from build123d import *

# Parameters (mm, degrees)
SKETCH1_W               = 40
SKETCH1_H               = 20
BOSS_EXTRUDE1_DEPTH     = 4
SKETCH2_W               = 10
SKETCH2_H               = 20
BOSS_EXTRUDE2_DEPTH     = 10
SKETCH3_R               = 1.5
CUT_EXTRUDE1_DEPTH      = 20
SKETCH4_R               = 1.5
CUT_EXTRUDE2_DEPTH      = 20
CUT_EXTRUDE3_DEPTH      = 43.242250662
CUT_EXTRUDE3_DEPTH_BACK = 20
SKETCH6_W               = 40
SKETCH6_H               = 20
BOSS_EXTRUDE3_DEPTH     = 4.5
CUT_EXTRUDE5_DEPTH      = 4.5
CUT_EXTRUDE6_DEPTH      = 14.5
SKETCH9_W               = 40
SKETCH9_H               = 20
CUT_EXTRUDE7_DEPTH      = 1.5


with BuildPart() as part:
    # Sketch1 → Boss-Extrude1 (new body)
    with BuildSketch(Plane(origin=(0, 0, 0), x_dir=(1, 0, 0), z_dir=(0, 1, 0))):
        with Locations((-14.473290255, 1.083337988)):
            Rectangle(SKETCH1_W, SKETCH1_H)
    extrude(amount=BOSS_EXTRUDE1_DEPTH)

    # Sketch2 → Boss-Extrude2 (add)
    with BuildSketch(Plane(origin=(0, 4, 0), x_dir=(1, 0, 0), z_dir=(0, 1, 0))):
        with Locations((-14.473290255, 1.083337988)):
            Rectangle(SKETCH2_W, SKETCH2_H)
    extrude(amount=BOSS_EXTRUDE2_DEPTH)

    # Sketch3 → Cut-Extrude1 (cut)
    with BuildSketch(Plane(origin=(-9.473290255, 0, 0), x_dir=(0, 0, -1), z_dir=(1, 0, 0))):
        with Locations((1.083337988, 9.951)):
            Circle(SKETCH3_R)
    extrude(amount=-CUT_EXTRUDE1_DEPTH, mode=Mode.SUBTRACT)

    # Sketch4 → Cut-Extrude2 (cut)
    with BuildSketch(Plane(origin=(0, 4, 0), x_dir=(1, 0, 0), z_dir=(0, 1, 0))):
        with BuildLine():
            ThreePointArc((-1.073290255, 2.283337988), (-3.173290255, 1.983337988), (-2.873290255, -0.116662012))
            Line((-2.873290255, -0.116662012), (-1.073290255, 2.283337988))
        make_face()
        with BuildLine():
            Line((-1.073290255, 2.283337988), (-2.873290255, -0.116662012))
            ThreePointArc((-2.873290255, -0.116662012), (-1.302469862, -0.258302799), (-0.473290255, 1.083337988))
            ThreePointArc((-0.473290255, 1.083337988), (-0.631649468, 1.754158381), (-1.073290255, 2.283337988))
        make_face()
        with Locations(Location((-26.973290255, 1.083337988, 0), (0, 0, 270))):
            Circle(SKETCH4_R)
    extrude(amount=-CUT_EXTRUDE2_DEPTH, mode=Mode.SUBTRACT)

    # Sketch5 → Cut-Extrude3 (cut, two sides)
    with BuildSketch(Plane.XY.offset(8.916662012)) as cut_extrude3_sk:
        Polygon((100.285190147, 4), (5.526709745, 4), (1.526709745, 4), (5.526709745, 0), (72.531073812, -67.004364067), (249.0428395, -135.999110287), (276.796955834, -64.99474622), align=None)
    extrude(amount=CUT_EXTRUDE3_DEPTH, mode=Mode.SUBTRACT)
    extrude(cut_extrude3_sk.sketch, amount=-CUT_EXTRUDE3_DEPTH_BACK, mode=Mode.SUBTRACT)

    # Sketch6 → Boss-Extrude3 (add)
    with BuildSketch(Plane.XZ):
        with Locations((-14.473290255, -1.083337988)):
            Rectangle(SKETCH6_W, SKETCH6_H)
    extrude(amount=BOSS_EXTRUDE3_DEPTH)

    # Sketch7 → Cut-Extrude5 (cut)
    with BuildSketch(Plane(origin=(0, 0, 0), x_dir=(1, 0, 0), z_dir=(0, 1, 0))):
        with BuildLine():
            ThreePointArc((-0.473290255, 1.083337988), (-1.973290255, 2.583337988), (-3.473290255, 1.083337988))
            Line((-3.473290255, 1.083337988), (-0.473290255, 1.083337988))
        make_face()
        with BuildLine():
            Line((-0.473290255, 1.083337988), (-3.473290255, 1.083337988))
            ThreePointArc((-3.473290255, 1.083337988), (-1.973290255, -0.416662012), (-0.473290255, 1.083337988))
        make_face()
    extrude(amount=-CUT_EXTRUDE5_DEPTH, mode=Mode.SUBTRACT)

    # Sketch8 → Cut-Extrude6 (cut)
    with BuildSketch(Plane(origin=(0, 4, 0), x_dir=(1, 0, 0), z_dir=(0, 1, 0))):
        with BuildLine():
            ThreePointArc((-25.473290255, 1.083337988), (-26.973290255, 2.583337988), (-28.473290255, 1.083337988))
            Line((-28.473290255, 1.083337988), (-25.473290255, 1.083337988))
        make_face()
        with BuildLine():
            Line((-25.473290255, 1.083337988), (-28.473290255, 1.083337988))
            ThreePointArc((-28.473290255, 1.083337988), (-26.973290255, -0.416662012), (-25.473290255, 1.083337988))
        make_face()
    extrude(amount=-CUT_EXTRUDE6_DEPTH, mode=Mode.SUBTRACT)

    # Sketch9 → Cut-Extrude7 (cut)
    with BuildSketch(Plane(origin=(0, -4.5, 0), x_dir=(-1, 0, 0), z_dir=(0, -1, 0))):
        with Locations((14.473290255, 1.083337988)):
            Rectangle(SKETCH9_W, SKETCH9_H)
    extrude(amount=-CUT_EXTRUDE7_DEPTH, mode=Mode.SUBTRACT)


solid = part.part
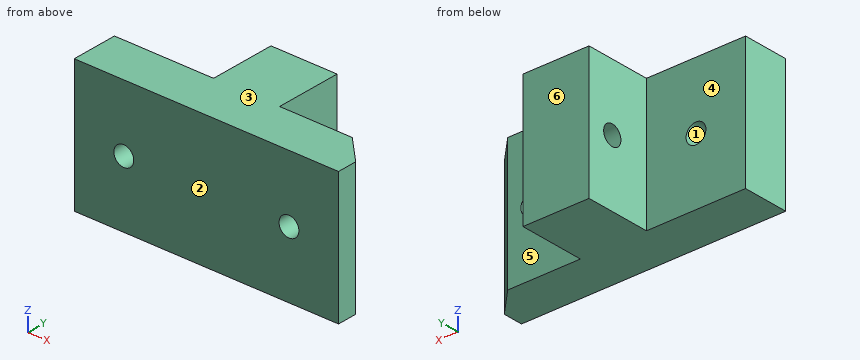
Source: CAD feature listing. Evaluate the final solid. Frame: model axes, mm. Face numbers are marked on the shaded views. A direction names the side the tool comes from. Round coordinates to 2 decimals unless told otherwise and drop trailing zeros. Loops run counter-clockwise (first coordinate to the right, second up) from the corner with the lowest first, then second, coordinate; pieces in that order, holes last.
Q1. Section A-A, the plane z = 6.5. Return loops of the section in (x, y).
Q2. Section D-D, the plane x = -8.5. Return loops of the section in (y, z), plus the area to 3 significant figures.
Q3. Ray query, line 1 (Y direction, x = -27.5, z = 8.25); line 2 (X direction, y = 6.5, z = 4); line 3 (Y direction, x = -15.5, z = -2). Return the intervals inside material, ascending.
Q4. Access query for the marked faces 4, 5 and 6. Directions: +Z, -Z, +X, -X, +Y, -Y. A direction counts if a zero-diameter tool reaches every point of the face in a straight line with its end or side. Return the directions, or none.
Q5. First-contact query: P1, Ø3, axis at y = 9.5, z = -4, coming from the -X side; P2, Ø3, axis at y = 5, z = -8, coming from the +X side; P3, Ø2.5, axis at x = -1.97, z = -1.08, coming from the +Y side; P4, Ø4.5, axis at x = -24, z = 3, coming from the +Y side. Flat tips, straight axial feed; report the tip coordinate or a pass-through.
Q6. Mould query, pull axis Z, two halves, no side actions, for the marked faces 1, 2 and 3. Classes: pulls with the +Z half, pulls with the -Z half, needs draft (parallel to the pull), parting line crosses it, or undercut.
Q7. Section C-C, the plane y = 6.5. Return loops of the section in (x, z), plus the area to 3 significant figures.
Q8. Section B-B, the plane x = -26.5. Return loops of the section in (y, z), plus the area to 3 significant figures.
Solutions:
1. outline: (-34.47, -3) - (5.53, -3) - (5.53, 0) - (1.53, 4) - (-9.47, 4) - (-9.47, 14) - (-19.47, 14) - (-19.47, 4) - (-34.47, 4) - close
2. outline: (-3, -11.08) - (4, -11.08) - (4, 8.92) - (-3, 8.92) - close
2. area: 140 mm2
3. line 1: y = -3 to 4
3. line 2: x = -19.47 to -9.47
3. line 3: y = -3 to 8.76, 11.14 to 14
4. face 4: +Z, -Z, -X, +Y
4. face 5: +Z, -Z, +X, +Y
4. face 6: +Z, -Z, +X, -X, +Y
5. P1: stops at x = -19.47
5. P2: stops at x = 2.03
5. P3: passes through
5. P4: stops at y = 4
6. face 1: undercut
6. face 2: needs draft
6. face 3: pulls with the +Z half
7. outline: (-19.47, -11.08) - (-9.47, -11.08) - (-9.47, 8.92) - (-19.47, 8.92) - close
7. area: 200 mm2
8. outline: (-3, -11.08) - (4, -11.08) - (4, -2.51) - (-3, -2.51) - close; (-3, 0.34) - (4, 0.34) - (4, 8.92) - (-3, 8.92) - close
8. area: 120 mm2
